Source: CAD feature listing. Evaluate the final solid. Frame: model axes, mm. A direction names the side the tool comes from. Round coordinates to 2 decimals unless told otherwise and drop trailing zeros. Loops run counter-clockwise (first coordinate to the right, second up) from the corner with the lowest first, then second, coordinate; pieces in that order, holes last. Notation, with made-up numbers: (-3, 87) -> (55, 87) arc R12 cw to (55, 104) -> close; hole circle Ø10 at (-39, 69.5). An arc over 180 degrees is marked (long way). Write item = value, one per line.
Autodesk Inventor part; units mm, degrees
ref_plane "YZ Plane" through (0, 0, 0) normal (1, 0, 0) x (0, 1, 0)
ref_plane "XZ Plane" through (0, 0, 0) normal (0, 1, 0) x (-1, 0, 0)
ref_plane "XY Plane" through (0, 0, 0) normal (0, 0, 1) x (1, 0, 0)
sketch "Sketch1" plane through (0, 0, 0) normal (0, 1, 0) x (-1, 0, 0)
  circle A0 centre (0, 0) radius 30
  circle A1 centre (0, 0) radius 25
  dimension "d0" = 60
  dimension "d1" = 50
extrude "Extrusion1" add sketch "Sketch1" against normal blind 1.5
sketch "Sketch2" plane through (0, -1.5, 0) normal (0, -1, 0) x (1, 0, 0)
  line L0 (-2, 28.5) -> (2, 28.5)
  line L1 (2, 28.5) -> (2, 26.5)
  line L2 (2, 26.5) -> (-2, 26.5)
  line L3 (-2, 26.5) -> (-2, 28.5)
  point P0 (0, 0)
  point P1 (0, 28.5)
  dimension "d4" = 2
  dimension "d5" = 26.5
  dimension "d6" = 4
extrude "Extrusion2" add sketch "Sketch2" along normal blind 0.75
pattern_circular "Circular Pattern1" count 15 over 360 about axis through (0, -10, 0) along (0, 1, 0) of "Extrusion2"
properties part number "fc18-097" material "Polypropylene"
1. Contact query for flat-ended pins moving along their axis: pin 1 Ø0.8 at (x, y) = (1, -2) entering from -Z; pin 2 Ø0.6 at (y, z) = (-2, 28) entering from +X; pin 3 Ø0.6 at (y, z) = (-2, 27) entering from -X. Output: stop coordinate, or through.
Evaluation:
pin_1 = 26.5
pin_2 = 2
pin_3 = -10.1
2. Section query D-D (x = 16). Return the cut outline in (y, z).
Evaluation:
outline = (-2.25, -23.6) -> (-1.5, -23.6) -> (-1.5, -25.38) -> (0, -25.38) -> (0, -19.21) -> (-1.5, -19.21) -> (-1.5, -21.13) -> (-2.25, -21.13) -> close; (-1.5, 19.21) -> (0, 19.21) -> (0, 25.38) -> (-1.5, 25.38) -> close
3. Section query A-A (x = 0). Return the cut outline in (y, z).
Evaluation:
outline = (-2.25, 26.5) -> (-1.5, 26.5) -> (-1.5, 25) -> (0, 25) -> (0, 30) -> (-1.5, 30) -> (-1.5, 28.5) -> (-2.25, 28.5) -> close; (-1.5, -30) -> (0, -30) -> (0, -25) -> (-1.5, -25) -> close
4. Set-up query: faces 1 (the face through (-21.2, -1.87, 19.05)), 2 (the face through (-22.96, -1.87, -13.23)), 3 (the face through (21.16, -1.87, 19.09)), 4 (the face through (24.696, -1.87, -14.226)), 5 (the face through (-19.11, -1.87, 19.9)). Return all of +Z, -Z, +X, -X, +Y, -Y with unobstructed straight access to the full face (end or side cutting, diameter ignored); none if empty.
Evaluation:
face_1 = +Z, -X, -Y
face_2 = -Y
face_3 = +Z, +X, -Y
face_4 = -Z, +X, -Y
face_5 = +Z, -Y
5. Section query B-B (z = 0). Return the cut outline in (x, y), then the cut area to 3 significant figures.
Evaluation:
outline = (-30, -1.5) -> (-25, -1.5) -> (-25, 0) -> (-30, 0) -> close; (25, -1.5) -> (30, -1.5) -> (30, 0) -> (25, 0) -> close
area = 15.0 mm²
6. Section query C-C (y = -1.1). Return the cut outline in (x, z).
Evaluation:
outline = circle Ø60 at (0, 0); hole circle Ø50 at (0, 0)
7. Line query: probe 1 along Z at (x, y) = (0, -0.8); probe 2 along Y at (x, z) = (-16.5, -24); probe 3 along X at (y, z) = (-1.4, 10). Output: solid intervals per line, ascending. Write a range as from..to.
Evaluation:
probe_1 = -30..-25, 25..30
probe_2 = -1.5..0
probe_3 = -28.28..-22.91, 22.91..28.28
8. Mould query, pull axis Z, two halves, no side actions, for faces 6 (the face through (-15.6, -1.87, -21.42)), 7 (the face through (-23.846, -0.74, 7.509)), 8 (the face through (27, -2.25, -3)). Classes: released by +Z, released by -Z, zero draft, split by the parting line, or undercut.
Evaluation:
face_6 = released by +Z
face_7 = undercut
face_8 = zero draft
